from build123d import *

# Parameters (mm, degrees)
SKETCH1_W           = 100
SKETCH1_H           = 35
BOSS_EXTRUDE1_DEPTH = 5
SKETCH2_R           = 1.6
CUT_EXTRUDE1_DEPTH  = 5
FILLET1_R           = 1


with BuildPart() as part:
    # Sketch1 → Boss-Extrude1 (new body)
    with BuildSketch(Plane.XY):
        Rectangle(SKETCH1_W, SKETCH1_H)
    extrude(amount=BOSS_EXTRUDE1_DEPTH)

    # Sketch2 → Cut-Extrude1 (cut)
    with BuildSketch(Plane.XY.offset(5)):
        with Locations((-46.5, 14)):
            Circle(SKETCH2_R)
        with Locations((-46.5, -14)):
            Circle(SKETCH2_R)
        with Locations((46.5, 14)):
            Circle(SKETCH2_R)
        with Locations((46.5, -14)):
            Circle(SKETCH2_R)
    extrude(amount=-CUT_EXTRUDE1_DEPTH, mode=Mode.SUBTRACT)

    # Fillet1
    fillet1_edges = [part.edges().sort_by_distance(p)[0] for p in [
        (50, 0, 5),
        (0, 17.5, 5),
        (-50, 0, 5),
        (0, -17.5, 5),
    ]]
    fillet(fillet1_edges, radius=FILLET1_R)


solid = part.part
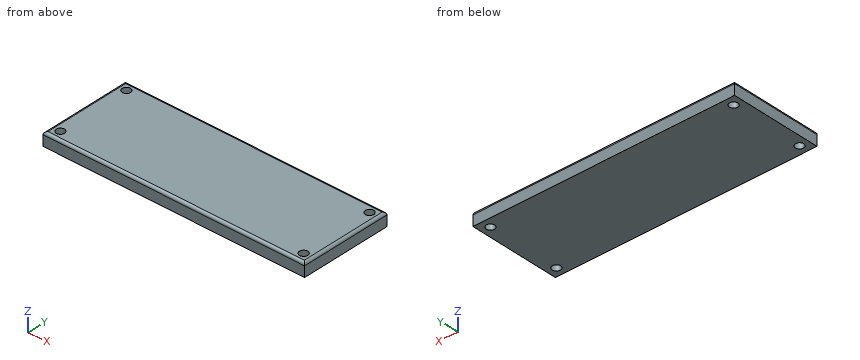
Geometry: final body of the model. Coordinates: model frame, mm. Coordinates: 2 decimals unless noted, no trailing zeros. Loops run counter-clockwise (first coordinate to the right, second up) from the corner with the lowest first, then second, coordinate; pieces in that order, holes last. Notation, with made-up numbers: (-8.5, 18) - (3.5, 18) arc R7 ccw to (3.5, 29) - close; hole circle Ø2 at (12.25, -6.5). An arc over 180 degrees is marked (long way). Put each result on its own line as item: value. Start each with the question number.
Q1. Cut plane B-B, the plane x = 46.5. Return loops of the section in (y, z).
Q2. Cut plane A-A, the plane y = 14. Return loops of the section in (x, z), and give its area (3 significant figures).
Q3. Line query: line 1 (Y direction, x = 46.5, z = 1.5); line 2 (X direction, y = 6, z = 4.05); line 3 (Y direction, x = -32, z = 4.25). Output: solid intervals per line, ascending.
Filled sheet:
1. outline: (-17.5, 0) - (-15.6, 0) - (-15.6, 5) - (-16.5, 5) arc R1 ccw to (-17.5, 4) - close; (-12.4, 0) - (12.4, 0) - (12.4, 5) - (-12.4, 5) - close; (15.6, 0) - (17.5, 0) - (17.5, 4) arc R1 ccw to (16.5, 5) - (15.6, 5) - close
2. outline: (-50, 0) - (-48.1, 0) - (-48.1, 5) - (-49, 5) arc R1 ccw to (-50, 4) - close; (-44.9, 0) - (44.9, 0) - (44.9, 5) - (-44.9, 5) - close; (48.1, 0) - (50, 0) - (50, 4) arc R1 ccw to (49, 5) - (48.1, 5) - close
2. area: 468 mm²
3. line 1: -17.5 to -15.6, -12.4 to 12.4, 15.6 to 17.5
3. line 2: -50 to 50
3. line 3: -17.47 to 17.47
